```python
from build123d import *

# Parameters (mm, degrees)
SKETCH1_W                  = 100
SKETCH1_H                  = 175
BOSS_EXTRUDE1_DEPTH        = 20
F_5_0_5_DIAMETER_HOLE1_D   = 5
F_12_0_12_DIAMETER_HOLE1_D = 12
F_20_0_20_DIAMETER_HOLE1_D = 20


with BuildPart() as part:
    # Sketch1 → Boss-Extrude1 (new body)
    with BuildSketch(Plane.XY):
        with Locations((50, 87.5)):
            Rectangle(SKETCH1_W, SKETCH1_H)
    extrude(amount=-BOSS_EXTRUDE1_DEPTH)

    # Ø5.0 (5) Diameter Hole1 (through all)
    with Locations(Plane.XY):
        with Locations((25, 145)):
            Hole(F_5_0_5_DIAMETER_HOLE1_D / 2)

    # Ø12.0 (12) Diameter Hole1 (through all)
    with Locations(Plane.XY):
        with Locations((50, 87.5)):
            Hole(F_12_0_12_DIAMETER_HOLE1_D / 2)

    # Ø20.0 (20) Diameter Hole1 (through all)
    with Locations(Plane.XY):
        with Locations((75, 30)):
            Hole(F_20_0_20_DIAMETER_HOLE1_D / 2)


solid = part.part
```
For this review, take the finished solid that the model builds, in its own axes (mm). Give positions to 0.01 mm unless a question says otherwise; leave off trailing zeros. Order: outer loops, then holes, each group sorted by start corner. A loop starts at its lowest first (then second) coordinate and runs counter-clockwise, first axis right, second up.
1) Wall thickness on line 1 (Y direction, x = 50, z = -6.5); line 2 (Y direction, x = 75, z = -11.25); line 3 (X direction, y = 145, z = -9.5): over which ranges is each line inside the solid? List them lowest first.
2) Insertion check: pin 1 (1.5 mm diameter, centred on x = 52.5, y = 93, fed in from +Z); pin 2 (12 mm diameter, centred on x = 75, y = 30, fed in from -Z). Each pin has a flat end and moves straight along its axis. Give the tip position at first contact, or say it passes through.
3) Take a section at C-C (z = -13.5). Give the boundary of the cut face in (x, y), then the cut area to 3 significant figures.
4) The part is to be moulded in two halves that separate along X. For faces 1 (the face through (49, 175, -10)), 2 (the face through (25.33, 147.48, -10.14)), 3 (the face through (50.78, 93.45, -10.14)), 4 (the face through (0, 86, -10)), say which applies: released by +X, released by -X, zero draft, split by the parting line, or undercut.
5) Take a section at B-B (x = 25). Give the boundary of the cut face in (y, z), then the cut area to 3 significant figures.
6) Take a section at A-A (y = 87.5). Give the boundary of the cut face in (x, z), then the cut area to 3 significant figures.
Derived:
1. line 1: y = 0 to 81.5, 93.5 to 175
1. line 2: y = 0 to 20, 40 to 175
1. line 3: x = 0 to 22.5, 27.5 to 100
2. pin 1: stops at z = 0
2. pin 2: passes through
3. outline: (0, 0) - (100, 0) - (100, 175) - (0, 175) - close; hole circle Ø5 at (25, 145); hole circle Ø12 at (50, 87.5); hole circle Ø20 at (75, 30)
3. area: 17,100 mm2
4. face 1: zero draft
4. face 2: undercut
4. face 3: undercut
4. face 4: released by -X
5. outline: (0, -20) - (142.5, -20) - (142.5, 0) - (0, 0) - close; (147.5, -20) - (175, -20) - (175, 0) - (147.5, 0) - close
5. area: 3,400 mm2
6. outline: (0, -20) - (44, -20) - (44, 0) - (0, 0) - close; (56, -20) - (100, -20) - (100, 0) - (56, 0) - close
6. area: 1,760 mm2
